Verification items for this drawing (mm, ordinates from the low corner). Round coordinates to 2 decimals unless told otherwise and drop trailing zeros. Write each loop counter-clockwise with the first axis right and the second up, starting at its lowest first coordinate (ties: lowest second). Pieces come first, ordered by that corner, then holes.
Item 1: Cross-section at A-A (y = 46.5). Enter the section's corners in (x, z).
Item 2: Cross-section at B-B (z = 2.2). State how many separate pieces and enclosed holes the cut face has, then the cut area to 3 significant figures.
Item 3: Depth check by flat-ended pin: P1, Ø1.5, axis at x = 26.5, z = 1.5, coming from the -Y side; P2, Ø1.2, axis at x = 1.5, z = 2, coming from the +Y side. Enter the tip coordinate at first touch or a pass-through.
Item 4: Cross-section at C-C (x = 8.5). Enter the section's corners in (y, z), then the cut area to 3 significant figures.
Item 5: Scan lines: probe 1 along Y at (x, z) = (40.5, 0.8); probe 2 along Y at (x, z) = (32.5, 0.1); probe 3 along X at (y, z) = (11, 2.05). Record each from-to range of solid material in increasing order.
Item 6: Cross-section at D-D (y = 26). Enter the section's corners in (x, z), then the cut area to 3 significant figures.
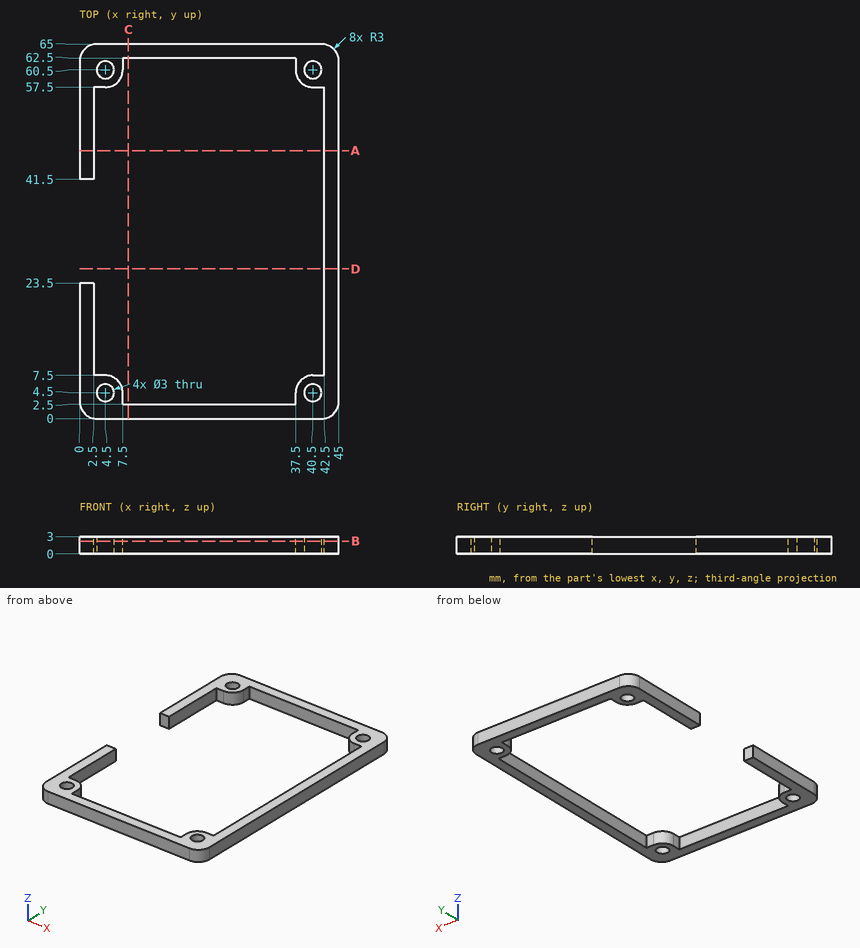
Resolved:
1. outline: (0, 0) - (2.5, 0) - (2.5, 3) - (0, 3) - close; (42.5, 0) - (45, 0) - (45, 3) - (42.5, 3) - close
2. separate pieces: 1
2. enclosed holes: 4
2. area: 536 mm2
3. P1: stops at y = 0
3. P2: stops at y = 64.86
4. outline: (0, 0) - (2.5, 0) - (2.5, 3) - (0, 3) - close; (62.5, 0) - (65, 0) - (65, 3) - (62.5, 3) - close
4. area: 15.0 mm2
5. probe 1: y = 0 to 3, 6 to 7.5, 57.5 to 59, 62 to 65
5. probe 2: y = 0 to 2.5, 62.5 to 65
5. probe 3: x = 0 to 2.5, 42.5 to 45
6. outline: (42.5, 0) - (45, 0) - (45, 3) - (42.5, 3) - close
6. area: 7.50 mm2
